Geometry check sheet. Reference: drawing and pictorial views, mm from the part's lowest x, y, z. Round coordinates to 2 decimals unless told otherwise and drop trailing zeros. Order: outer loops, then holes, each group sorted by start corner. A loop starts at its lowest first (then second) coordinate and runs counter-clockwise, first axis right, second up.
(1) Sectioned sample at C-C, the plane x = 16.5. Count the separate pieces of the cut face and the enclosed holes in it, and give its area (3 significant figures).
(2) Mould release check, pull along X, two halves, no side actions. Record for the marked faces 1, 2 and 3: released by +X, released by -X, zero draft, split by the parting line, or undercut.
(3) Thickness scan on probe 1 along Z at (x, y) = (16.5, 25); probe 2 along X at (y, z) = (25, 5) (1 decimal); probe 3 along X at (y, z) = (13.5, 3.5) (1 decimal). Record the ranges inside material, lowest first.
(4) Sectioned sample at B-B, the plane y = 23. Enter the section's corners in (x, z) (1 decimal), and give its area (3 significant figures).
(5) Depth check by flat-ended pin: pin 1 (2.5 mm diameter, centred on y = 12.7, z = 4.76, fed in from +X); pin 2 (3 mm diameter, centred on y = 34.92, z = 4.76, fed in from -X); pin 3 (2.5 mm diameter, centred on x = 14.5, y = 12.5, fed in from -Z) (1 decimal). Enter the tip coordinate at first touch or a pass-through.
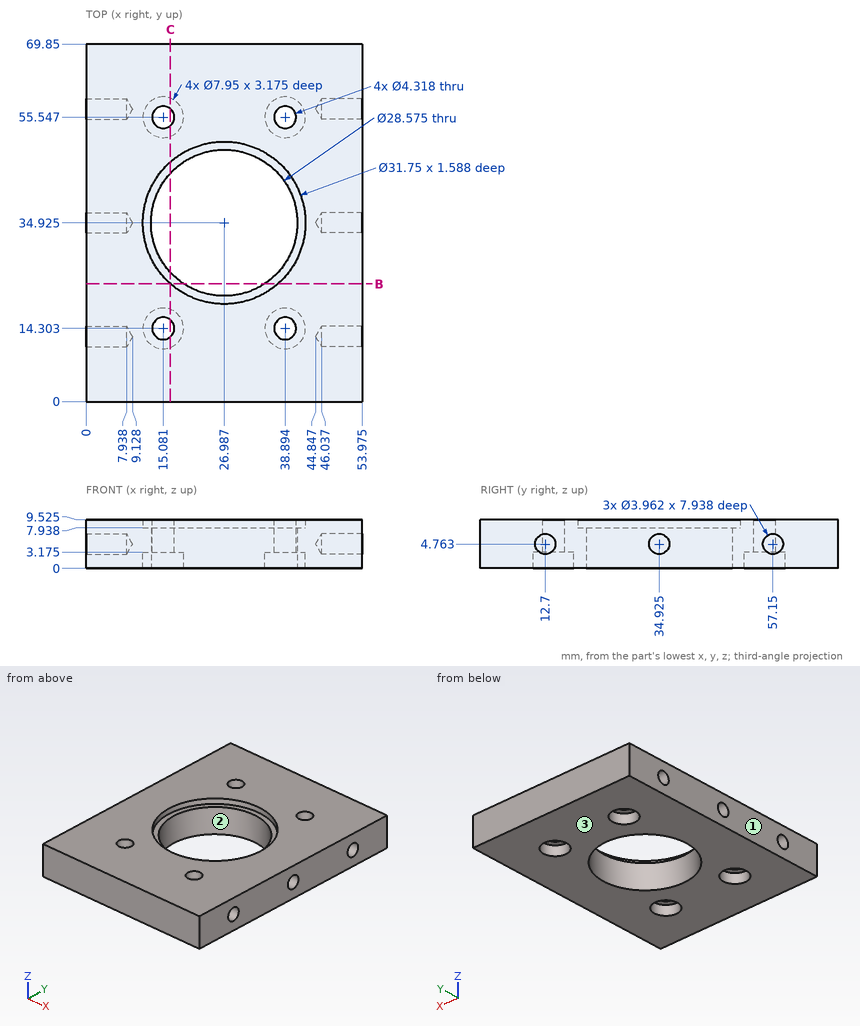
Derived:
1. separate pieces: 4
1. enclosed holes: 0
1. area: 385 mm2
2. face 1: released by -X
2. face 2: undercut
2. face 3: zero draft
3. probe 1: z = 0 to 7.94
3. probe 2: x = 0 to 16.7, 37.3 to 54
3. probe 3: x = 8.2 to 13.1, 17.1 to 36.9, 40.9 to 45.7
4. outline: (0, 0) - (19.1, 0) - (19.1, 7.9) - (16.5, 7.9) - (16.5, 9.5) - (0, 9.5) - close; (34.9, 0) - (54, 0) - (54, 9.5) - (37.5, 9.5) - (37.5, 7.9) - (34.9, 7.9) - close
4. area: 356 mm2
5. pin 1: stops at x = 45.6
5. pin 2: stops at x = 8.22
5. pin 3: stops at z = 3.2
